Geometry: final body of the model. Coordinates: model frame, mm. Face numbers are marked on the shaded views. A direction names the side the tool comes from. Coordinates: 2 decimals unless noted, no trailing zeros. Write each loop counter-clockwise with the first axis right and the second up, starting at its lowest first coordinate (ties: lowest second). Pieces come first, ordered by that corner, then holes.
from build123d import *

# Parameters (mm, degrees)
EXTRUDE_1_DEPTH = 2
SKETCH_2_R      = 9
EXTRUDE_2_DEPTH = 23
SKETCH_4_R      = 10
EXTRUDE_3_DEPTH = 5


with BuildPart() as part:
    # 草图1 → 凸台-拉伸1 (new body)
    with BuildSketch(Plane(origin=(0, 0, 0), x_dir=(1, 0, 0), z_dir=(0, 1, 0))):
        with BuildLine():
            Line((17.5, -11.5), (2.5, -11.5))
            ThreePointArc((2.5, -11.5), (1.767766953, -13.267766953), (0, -14))
            Line((0, -14), (0, -23))
            Line((0, -23), (20, -23))
            Line((20, -23), (20, -14))
            ThreePointArc((20, -14), (18.232233047, -13.267766953), (17.5, -11.5))
        make_face()
        with BuildLine():
            ThreePointArc((0, -9), (1.767766953, -9.732233047), (2.5, -11.5))
            Line((2.5, -11.5), (17.5, -11.5))
            ThreePointArc((17.5, -11.5), (18.232233047, -9.732233047), (20, -9))
            Line((20, -9), (20, 0))
            Line((20, 0), (0, 0))
            Line((0, 0), (0, -9))
        make_face()
        with BuildLine():
            ThreePointArc((0, -10.5), (0.707106781, -10.792893219), (1, -11.5))
            Line((1, -11.5), (2.5, -11.5))
            ThreePointArc((2.5, -11.5), (1.767766953, -9.732233047), (0, -9))
            Line((0, -9), (0, -10.5))
        make_face()
        with BuildLine():
            Line((2.5, -11.5), (1, -11.5))
            ThreePointArc((1, -11.5), (0.707106781, -12.207106781), (0, -12.5))
            Line((0, -12.5), (0, -14))
            ThreePointArc((0, -14), (1.767766953, -13.267766953), (2.5, -11.5))
        make_face()
        with BuildLine():
            ThreePointArc((0, -12.5), (-1, -11.5), (0, -10.5))
            Line((0, -10.5), (0, -9))
            ThreePointArc((0, -9), (-2.5, -11.5), (0, -14))
            Line((0, -14), (0, -12.5))
        make_face()
        with BuildLine():
            ThreePointArc((20, -9), (18.232233047, -9.732233047), (17.5, -11.5))
            Line((17.5, -11.5), (19, -11.5))
            ThreePointArc((19, -11.5), (19.292893219, -10.792893219), (20, -10.5))
            Line((20, -10.5), (20, -9))
        make_face()
        with BuildLine():
            Line((19, -11.5), (17.5, -11.5))
            ThreePointArc((17.5, -11.5), (18.232233047, -13.267766953), (20, -14))
            Line((20, -14), (20, -12.5))
            ThreePointArc((20, -12.5), (19.292893219, -12.207106781), (19, -11.5))
        make_face()
        with BuildLine():
            ThreePointArc((22.5, -11.5), (21.767766953, -9.732233047), (20, -9))
            Line((20, -9), (20, -10.5))
            ThreePointArc((20, -10.5), (20.707106781, -10.792893219), (21, -11.5))
            ThreePointArc((21, -11.5), (20.707106781, -12.207106781), (20, -12.5))
            Line((20, -12.5), (20, -14))
            ThreePointArc((20, -14), (21.767766953, -13.267766953), (22.5, -11.5))
        make_face()
    extrude(amount=EXTRUDE_1_DEPTH)

    # 草图2 → 凸台-拉伸2 (add)
    with BuildSketch(Plane(origin=(0, 2, 0), x_dir=(1, 0, 0), z_dir=(0, 1, 0))):
        with Locations(Location((10.062202952, -11.571533395, 0), (0, 0, 2.511658154))):
            Circle(SKETCH_2_R)
    extrude(amount=EXTRUDE_2_DEPTH)

    # 草图4 → 凸台-拉伸3 (add)
    with BuildSketch(Plane(origin=(0, 25, 0), x_dir=(1, 0, 0), z_dir=(0, 1, 0))):
        with Locations(Location((10.062202952, -11.571533395, 0), (0, 0, 270))):
            Circle(SKETCH_4_R)
    extrude(amount=EXTRUDE_3_DEPTH)


solid = part.part
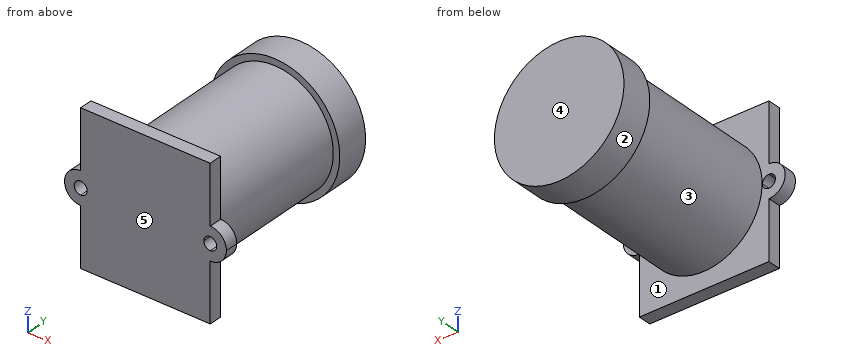
Item 1: Pin query (flat end, axial travel): pin 1 (5 mm diameter, centred on x = 6, y = 12, fed in from -Z); pin 2 (8 mm diameter, centred on x = 7.5, z = 19.5, fed in from -Y); pin 3 (1 mm diameter, centred on y = 1, z = 19, fed in from -X); pin 4 (10 mm diameter, centred on y = 22.5, z = 6, fed in from +X). Return the tip coordinate at first contact, or that it passes through.
Derived:
pin 1: stops at z = 2.71
pin 2: stops at y = 0
pin 3: stops at x = 0
pin 4: stops at x = 19.98
Item 2: Section C-C, the plane x = 4. Output: boundary loops of the cut face in (y, z).
Derived:
outline: (0, 0) - (2, 0) - (2, 4.92) - (25, 4.92) - (25, 3.62) - (30, 3.62) - (30, 19.52) - (25, 19.52) - (25, 18.22) - (2, 18.22) - (2, 23) - (0, 23) - close
Item 3: Set-up query: the marked faces 1 and 2. Return all of +Z, -Z, +X, -X, +Y, -Y with unobstructed straight access to the full face (end or side cutting, diameter ignored); none if empty.
Derived:
face 1: none
face 2: +Y
Item 4: Section B-B, the plane z = 3. Output: boundary loops of the cut face in (x, y), plus the area to 3 significant figures.
Derived:
outline: (0, 0) - (20, 0) - (20, 2) - (12.81, 2) - (12.81, 25) - (15.21, 25) - (15.21, 30) - (4.91, 30) - (4.91, 25) - (7.32, 25) - (7.32, 2) - (0, 2) - close
area: 218 mm2
Item 5: Pull-direction query (Y, two-part tool) for the marked faces 3, 4 and 5; classes: released by +Y, released by -Y, zero draft, split by the parting line, or undercut.
Derived:
face 3: undercut
face 4: released by +Y
face 5: released by -Y
Item 6: Section D-D, the plane y = 19.75. Output: boundary loops of the cut face in (x, z).
Derived:
outline: circle Ø18 at (10.06, 11.57)
Item 7: Section A-A, the plane x = 0.5. Output: boundary loops of the cut face in (y, z), plus the area to 3 significant figures.
Derived:
outline: (0, 0) - (2, 0) - (2, 10.63) - (0, 10.63) - close; (0, 12.37) - (2, 12.37) - (2, 23) - (0, 23) - close; (25, 8.65) - (30, 8.65) - (30, 14.5) - (25, 14.5) - close
area: 71.8 mm2
Item 8: Material intervals for probe 1 along Y at (x, z) = (13.75, 1.5); probe 2 along Y at (x, z) = (19, 8.75); probe 3 along Z at (x, y) = (14.25, 24), sorted ascending.
Derived:
probe 1: y = 0 to 2
probe 2: y = 0 to 2, 25 to 30
probe 3: z = 3.61 to 19.54
